Check sheet for the drawn part. Datum: minimum x, y, z corner. Units: mm. A direction names the side the tool comes from. Coordinates: 2 decimals unless noted, no trailing zeros. Write each loop counter-clockwise with the first axis right and the second up, starting at its lowest first coordinate (ties: lowest second). Pieces come first, ordered by that corner, then holes. Notation, with made-up numbers: M 18.5,86 L 70.5,86 A26 ccw 70.5,103 Z; hole C 74,-14.5 d9. An arc over 180 degrees is marked long. Answer in a Markdown table with one row per item.
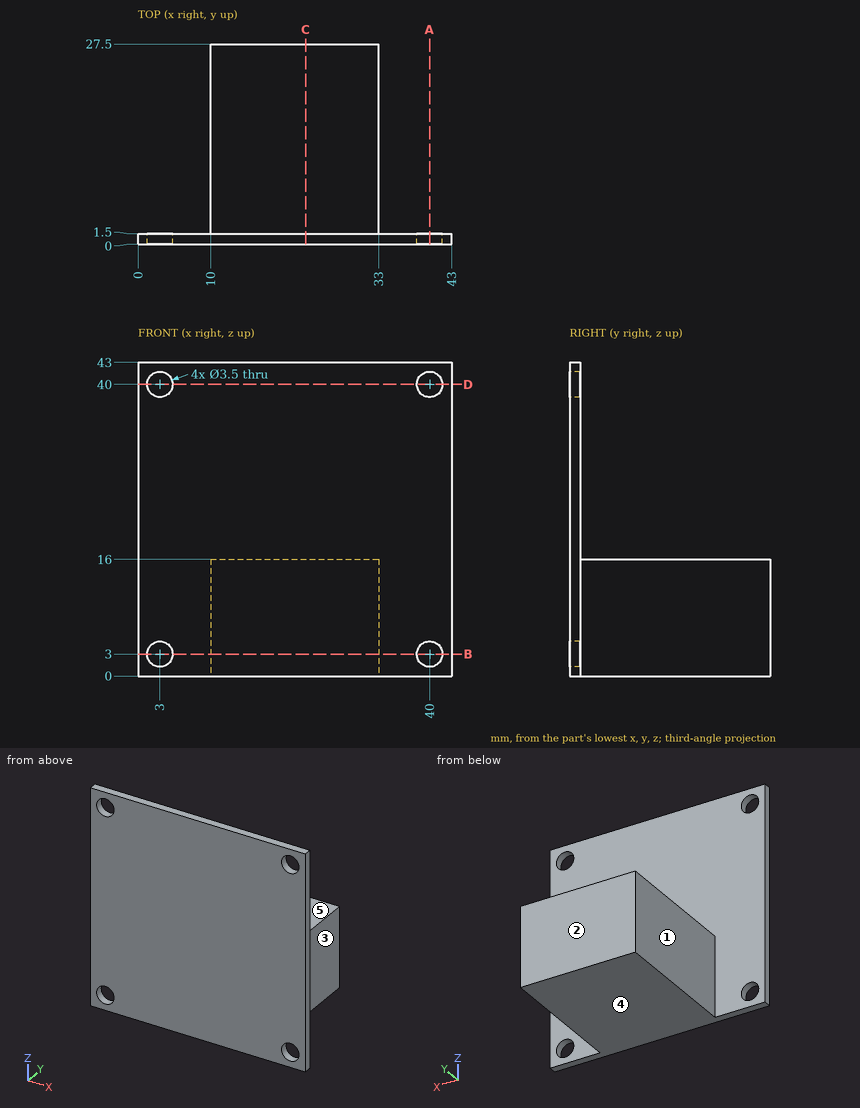
1) Tool access check on the marked faces 1, 2, 3, 4 and 5. Record the directions out of +Z, -Z, +X, -X, +Y, -Y that give a thin tool (end or side, any length) a straight path to the whole face; none if there is none.
Response values:
| item | result |
|---|---|
| face 1 | +Z, -Z, -X, +Y |
| face 2 | +Z, -Z, +X, -X, +Y |
| face 3 | +Z, -Z, +X, +Y |
| face 4 | -Z, +X, -X, +Y, -Y |
| face 5 | +Z, +X, -X, +Y |
2) Sectioned sample at D-D (z = 40). Record the cut outline in (x, y).
Response values:
| item | result |
|---|---|
| outline | M 0,0 L 1.25,0 L 1.25,1.5 L 0,1.5 Z; M 4.75,0 L 38.25,0 L 38.25,1.5 L 4.75,1.5 Z; M 41.75,0 L 43,0 L 43,1.5 L 41.75,1.5 Z |
3) Thickness scan on L1, parallel to X at y = 1, z = 3; L2, parallel to Z at x = 13.5, y = 2; L3, parallel to Y at x = 26, z = 26.5. Record the ranges inside material, lowest first. Write a range as [from, to].
Response values:
| item | result |
|---|---|
| L1 | x = [0, 1.25], [4.75, 38.25], [41.75, 43] |
| L2 | z = [0, 16] |
| L3 | y = [0, 1.5] |
4) Sectioned sample at C-C (x = 23). Record the cut outline in (y, z), then the cut area to 4 significant figures.
Response values:
| item | result |
|---|---|
| outline | M 0,0 L 27.5,0 L 27.5,16 L 1.5,16 L 1.5,43 L 0,43 Z |
| area | 480.5 mm² |
5) Depth check by flat-ended pin: pin 1 (3 mm diameter, centred on y = 16, z = 12.5, fed in from +X); pin 2 (5.5 mm diameter, centred on x = 3, z = 3, fed in from -Y); pin 3 (2 mm diameter, centred on x = 22.5, y = 3, fed in from +Z); pin 4 (1.5 mm diameter, centred on x = 21.5, z = 20.5, fed in from +Y). Enter the tip coordinate at first touch or a pass-through.
Response values:
| item | result |
|---|---|
| pin 1 | stops at x = 33 |
| pin 2 | stops at y = 0 |
| pin 3 | stops at z = 16 |
| pin 4 | stops at y = 1.5 |
6) Sectioned sample at B-B (z = 3). Record the cut outline in (x, y).
Response values:
| item | result |
|---|---|
| outline | M 0,0 L 1.25,0 L 1.25,1.5 L 0,1.5 Z; M 4.75,0 L 38.25,0 L 38.25,1.5 L 33,1.5 L 33,27.5 L 10,27.5 L 10,1.5 L 4.75,1.5 Z; M 41.75,0 L 43,0 L 43,1.5 L 41.75,1.5 Z |
7) Sectioned sample at A-A (x = 40). Record the cut outline in (y, z), then the cut area to 3 significant figures.
Response values:
| item | result |
|---|---|
| outline | M 0,0 L 1.5,0 L 1.5,1.25 L 0,1.25 Z; M 0,4.75 L 1.5,4.75 L 1.5,38.25 L 0,38.25 Z; M 0,41.75 L 1.5,41.75 L 1.5,43 L 0,43 Z |
| area | 54.0 mm² |
